Geometry: final body of the model. Coordinates: model frame, mm. A direction names the side the tool comes from. Give positions to 0.01 mm unless a question says otherwise; leave off trailing zeros. Write each loop counter-clockwise with the first axis right and the second up, starting at its lowest first coordinate (ties: lowest second). Pieces come first, ordered by that corner, then holes. Notation, with made-up numbers: (53, 69) - (90, 69) arc R24 ccw to (90, 94) - close; hole circle Ø4 at (0, 55). An arc over 180 degrees is marked (long way). Use CSV: the item, a comma, the result in double quotes. Start each with the question number.
(1) Section B-B on z = -15.5. Output: boundary loops of the cut face in (x, y), and give its area (3 significant figures).
(2) First-contact query: pin 1 Ø9 at (x, y) = (-5, -10) entering from -Z; pin 2 Ø4 at (x, z) = (-12.5, -15) entering from +Y; pin 3 Ø1.5 at (x, z) = (16, 16) entering from +Y. Flat tips, straight axial feed; report the tip coordinate or a pass-through.
(3) Draft query along X for faces 4 (the flat face through (-15, 1, -16)), 5 (the flat face through (16, 1, 15)), 6 (the flat face through (0, -9, 20.5)), 7 (the flat face through (-19, 4, 19)). Return one class per face: released by +X, released by -X, zero draft, split by the parting line, or undercut.
(4) Reachability of faces 1 (the cylindrical face through (-10.74, 8.99, -2.38)), 2 (the flat face through (17, -9, -18)), 3 (the flat face through (-17, -9, 18)) from +Z, -Z, +X, -X, +Y, -Y: full face, straight path, thin tool, end or side. Return the list, or none.
(5) Line query: probe 1 along X at (y, z) = (4, 15.5); probe 2 along X at (y, z) = (6, -15); probe 3 along Y at (x, z) = (-2.5, 5.5). Output: solid intervals per line, ascending. Write a range as [from, to].
(6) Section C-C on x = -12. Output: boundary loops of the cut face in (y, z), and give its area (3 significant figures).
(7) Section A-A on y = -13.5. Output: boundary loops of the cut face in (x, z).
(8) Section D-D on y = -22. Output: boundary loops of the cut face in (x, z), and give its area (3 significant figures).
from build123d import *

# Parameters (mm, degrees)
SKETCH1_W           = 42
SKETCH1_H           = 42
BOSS_EXTRUDE1_DEPTH = 8
LPATTERN2_COUNT     = 2
LPATTERN2_PITCH     = 26
BOSS_EXTRUDE4_REACH = 41.472
SKETCH5_W           = 41
SKETCH5_H           = 41
CHAMFER2_SIZE       = 6
CHAMFER1_SIZE       = 4
SKETCH2_R           = 11
BOSS_EXTRUDE2_DEPTH = 2
SKETCH3_R           = 2.5
BOSS_EXTRUDE3_DEPTH = 22
SKETCH6_R           = 1.5
CUT_EXTRUDE1_DEPTH  = 7


with BuildPart() as part:
    # Sketch1 → Boss-Extrude1 (new body)
    with BuildSketch(Plane(origin=(0, 0, 0), x_dir=(1, 0, 0), z_dir=(0, 1, 0))):
        Rectangle(SKETCH1_W, SKETCH1_H)
    extrude(amount=BOSS_EXTRUDE1_DEPTH)


with BuildPart() as lpattern2_1:
    # LPattern2: pattern copy
    add(part.part.moved(Location(Vector(0, -1, 0) * (1 * LPATTERN2_PITCH))))

    # Sketch5 → Boss-Extrude4 (add, up to next)
    with BuildSketch(Plane.XZ, mode=Mode.PRIVATE) as boss_extrude4_sk1:
        Rectangle(SKETCH5_W, SKETCH5_H)
    boss_extrude4_tool1 = extrude(boss_extrude4_sk1.sketch, amount=BOSS_EXTRUDE4_REACH, mode=Mode.PRIVATE) - lpattern2_1.part

    add(part.part)  # Boss-Extrude4 merges part
    add(boss_extrude4_tool1.solids().sort_by_distance((0, 0, 0))[0])

    # Chamfer2
    chamfer2_edges = [lpattern2_1.edges().sort_by_distance(p)[0] for p in [
        (20.5, -9, 20.5),
        (-20.5, -9, 20.5),
        (-20.5, -9, -20.5),
        (20.5, -9, -20.5),
    ]]
    chamfer(chamfer2_edges, length=CHAMFER2_SIZE)

    # Chamfer1
    chamfer1_edges = [lpattern2_1.edges().sort_by_distance(p)[0] for p in [
        (-21, -22, -21),
        (-21, -22, 21),
        (21, -22, 21),
        (21, -22, -21),
        (-21, 4, -21),
        (21, 4, -21),
        (21, 4, 21),
        (-21, 4, 21),
    ]]
    chamfer(chamfer1_edges, length=CHAMFER1_SIZE)

    # Sketch2 → Boss-Extrude2 (add)
    with BuildSketch(Plane(origin=(0, 8, 0), x_dir=(1, 0, 0), z_dir=(0, 1, 0))):
        with Locations(Location((0, 0, 0), (0, 0, 270))):
            Circle(SKETCH2_R)
    extrude(amount=BOSS_EXTRUDE2_DEPTH)

    # Sketch3 → Boss-Extrude3 (add)
    with BuildSketch(Plane(origin=(0, 10, 0), x_dir=(1, 0, 0), z_dir=(0, 1, 0))):
        with Locations(Location((0, 0, 0), (0, 0, 270))):
            Circle(SKETCH3_R)
    extrude(amount=BOSS_EXTRUDE3_DEPTH)

    # Sketch6 → Cut-Extrude1 (cut)
    with BuildSketch(Plane(origin=(0, 8, 0), x_dir=(1, 0, 0), z_dir=(0, 1, 0))):
        with Locations(Location((-15.5, 15.5, 0), (0, 0, 270))):
            Circle(SKETCH6_R)
        with Locations(Location((15.5, 15.5, 0), (0, 0, 270))):
            Circle(SKETCH6_R)
        with Locations(Location((15.5, -15.5, 0), (0, 0, 270))):
            Circle(SKETCH6_R)
        with Locations(Location((-15.5, -15.5, 0), (0, 0, 270))):
            Circle(SKETCH6_R)
    extrude(amount=-CUT_EXTRUDE1_DEPTH, mode=Mode.SUBTRACT)


solid = lpattern2_1.part
Check values:
1,outline,"(-21, -26) - (21, -26) - (21, -18) - (19.5, -18) - (19.5, 0) - (21, 0) - (21, 8) - (17, 8) - (17, 1) - (14, 1) - (14, 8) - (-14, 8) - (-14, 1) - (-17, 1) - (-17, 8) - (-21, 8) - (-21, 0) - (-19.5, 0) - (-19.5, -18) - (-21, -18) - close"
1,area,"1,330 mm²"
2,pin 1,"stops at z = -20.5"
2,pin 2,"stops at y = 8"
2,pin 3,"stops at y = 1"
3,face 4,"undercut"
3,face 5,"undercut"
3,face 6,"zero draft"
3,face 7,"released by -X"
4,face 1,"+Y"
4,face 2,"-Z, +X"
4,face 3,"+Z, -X"
5,probe 1,"x = [-21, -17], [-14, 14], [17, 21]"
5,probe 2,"x = [-21, -16.91], [-14.09, 14.09], [16.91, 21]"
5,probe 3,"y = [-26, 10]"
6,outline,"(-26, -21) - (-18, -21) - (-18, -20.5) - (0, -20.5) - (0, -21) - (8, -21) - (8, 21) - (0, 21) - (0, 20.5) - (-18, 20.5) - (-18, 21) - (-26, 21) - close"
6,area,"1,410 mm²"
7,outline,"(-20.5, -14.5) - (-14.5, -20.5) - (14.5, -20.5) - (20.5, -14.5) - (20.5, 14.5) - (14.5, 20.5) - (-14.5, 20.5) - (-20.5, 14.5) - close"
8,outline,"(-21, -17) - (-17, -21) - (17, -21) - (21, -17) - (21, 17) - (17, 21) - (-17, 21) - (-21, 17) - close"
8,area,"1,730 mm²"
